Geometry: final body of the model. Coordinates: model frame, mm. Coordinates: 2 decimals unless noted, no trailing zeros. Write each loop counter-clockwise with the first axis right and the second up, starting at its lowest first coordinate (ties: lowest second). Pieces come first, ordered by that corner, then holes. Notation, with made-up numbers: (-19, 44.25) - (22, 44.25) arc R32 cw to (22, 81.25) - close; hole circle Ø6 at (51.5, 54.5). An arc over 180 degrees is marked (long way). Put each result on its own line as item: value.
Autodesk Inventor part; units mm, degrees
ref_plane "YZ Plane" through (0, 0, 0) normal (1, 0, 0) x (0, 1, 0)
ref_plane "XZ Plane" through (0, 0, 0) normal (0, 1, 0) x (-1, 0, 0)
ref_plane "XY Plane" through (0, 0, 0) normal (0, 0, 1) x (1, 0, 0)
sketch "Sketch1" plane through (0, 0, 0) normal (0, 0, 1) x (1, 0, 0)
  line L0 (-114.3, 77.8543) -> (-127, 77.8543)
  line L1 (-127, 77.8543) -> (-163.2323, 36.0005)
  arc A0 (-163.2323, 36.0005) -> (-215.9, -105.3078) centre (0, -105.3078) ccw
  line L2 (-152.4, -105.3078) -> (-215.9, -105.3078)
  arc A1 (152.4, -105.3078) -> (-152.4, -105.3078) centre (0, -105.3078) ccw
  line L3 (215.9, -105.3078) -> (152.4, -105.3078)
  arc A2 (215.9, -105.3078) -> (163.2323, 36.0005) centre (0, -105.3078) ccw
  line L4 (163.2323, 36.0005) -> (127, 77.8543)
  line L5 (127, 77.8543) -> (114.3, 77.8543)
  line L6 (114.3, 77.8543) -> (114.3, 90.5543)
  line L7 (114.3, 90.5543) -> (46.5518, 105.5138)
  arc A3 (46.5518, 105.5138) -> (-46.5518, 105.5138) centre (0, -105.3078) ccw
  line L8 (-46.5518, 105.5138) -> (-114.3, 90.5543)
  line L9 (-114.3, 90.5543) -> (-114.3, 77.8543)
  circle A4 centre (-174.6359, -42.9949) radius 3.302
  circle A5 centre (-181.5133, -67.4461) radius 3.302
  circle A6 centre (-184.9846, -92.6078) radius 3.302
  circle A7 centre (-12.7, 63.1241) radius 3.302
  circle A8 centre (-37.8617, 76.2055) radius 3.302
  circle A9 centre (-62.0706, 51.784) radius 3.302
  circle A10 centre (12.7, 63.1241) radius 3.302
  circle A11 centre (62.0706, 51.784) radius 3.302
  circle A12 centre (62.3129, 69.3281) radius 3.302
  circle A13 centre (174.6359, -42.9949) radius 3.302
  circle A14 centre (164.6231, -67.4949) radius 3.302
  circle A15 centre (181.5133, -67.4461) radius 3.302
  circle A16 centre (184.9846, -92.6078) radius 3.302
  circle A17 centre (168.4319, -92.6078) radius 3.302
  circle A18 centre (157.0918, -43.2372) radius 3.302
  circle A19 centre (37.8617, 76.2055) radius 3.302
  circle A20 centre (37.8128, 59.3154) radius 3.302
  circle A21 centre (12.7, 79.6768) radius 3.302
  circle A22 centre (-62.3129, 69.3281) radius 3.302
  circle A23 centre (-37.8128, 59.3154) radius 3.302
  circle A24 centre (-12.7, 79.6768) radius 3.302
  circle A25 centre (-168.4319, -92.6078) radius 3.302
  circle A26 centre (-164.6231, -67.4949) radius 3.302
  circle A27 centre (-157.0918, -43.2372) radius 3.302
  line L10 (-127, 143.7166) -> (-127, -105.3078)
  line L11 (-127, -21.0655) -> (-127, 108.4537)
  line L12 (-142.24, -21.0655) -> (-142.24, 38.6612) construction
  circle A28 centre (-142.24, -7.2274) radius 3.302
  circle A29 centre (-142.24, 18.1726) radius 3.302
  line L13 (-157.48, -21.0655) -> (-157.48, 42.6453)
  line L14 (-127, -21.0655) -> (-157.48, -21.0655)
  line L15 (-127, 108.4537) -> (-131.3752, 105.9825)
  line L16 (-143.2518, 91.0321) -> (-157.48, 42.6453)
  arc A30 (-131.3752, 105.9825) -> (-143.2518, 91.0321) centre (-118.8834, 83.8665) ccw
  circle A31 centre (142.24, 14.8706) radius 3.302
  circle A32 centre (-142.24, 14.8706) radius 3.302
  circle A33 centre (-142.24, -10.5294) radius 3.302
  circle A34 centre (142.24, -10.5294) radius 3.302
  point P0 (0, 0)
  dimension "d1" = 6.604
  dimension "d2" = 6.604
  dimension "d3" = 25.4
  dimension "d6" = 15.24
  dimension "d7" = 15.24
  dimension "d8" = 25.4
extrude "Extrusion1" add sketch "Sketch1" along normal blind 3.175 contours L10 L14 L13 L1 | L1 L16 A30 L15 L10 | A28 A33 | A29 A32 picked at (-142.4059, -12.7065) picked at (-142.4059, 12.6935)
sketch "Sketch2" plane through (0, 0, 0) normal (0, 0, -1) x (-1, 0, 0)
  line L0 (127, -21.0655) -> (127, 108.4537)
  line L1 (157.48, 42.6453) -> (157.48, -21.0655)
  line L2 (127, -21.0655) -> (157.48, -21.0655)
  line L3 (157.48, -21.0655) -> (157.48, -15.2234)
  line L4 (157.48, -15.2234) -> (127, -15.2234)
  line L5 (127, -15.2234) -> (127, -21.0655)
  point P0 (0, 0)
extrude "Extrusion2" cut sketch "Sketch2" against normal blind 25.4
properties part number "16in coil holder plate" material "UHMW, Black"
1. Ray query, probe 1 along Y at (x, z) = (-142.24, 1.45); probe 2 along Y at (x, z) = (-140, 0.75); probe 3 along X at (y, z) = (75.5, 0.8). Return the intervals inside material, ascending. Write a range as from..to.
Answer below:
probe 1: y = -15.22..-10.53, -3.93..14.87, 21.47..93.85
probe 2: y = -15.22..-9.65, -4.8..15.75, 20.6..97.98
probe 3: x = -147.82..-127
2. Mould query, pull axis X, two halves, no side actions, for faces 1 (the flat face through (-127, 47, 2)), 2 (the cylindrical face through (-145.54, 18.03, 1.57)), 3 (the flat face through (-142, -15.223, 2)), 4 (the flat face through (-129.157, 107.235, 1.565)). Classes: +X half, -X half, draft (parallel to the pull), parting line (faces both ways), or undercut.
Answer below:
face 1: +X half
face 2: undercut
face 3: draft
face 4: -X half
3. Section query A-A (z = 1.3). Return loops of the section in (x, y).
Answer below:
outline: (-157.48, -15.22) - (-127, -15.22) - (-127, 108.45) - (-131.38, 105.98) arc R25.4 ccw to (-143.25, 91.03) - (-157.48, 42.65) - close; hole circle Ø6.6 at (-142.24, -7.23); hole circle Ø6.6 at (-142.24, 18.17)
4. Section query B-B (y = 71). Return loops of the section in (x, z) (3 decimals), then the cut area to 3 significant figures.
Answer below:
outline: (-149.142, 0) - (-127, 0) - (-127, 3.175) - (-149.142, 3.175) - close
area: 70.3 mm²
5. Section query C-C (x = -147). Return loops of the section in (y, z) (3 decimals).
Answer below:
outline: (-15.223, 0) - (78.285, 0) - (78.285, 3.175) - (-15.223, 3.175) - close
6. Pin query (flat end, axial travel): pin 1 Ø7.5 at (x, y) = (-142.24, -7.23) entering from +Z (3 decimals); pin 2 Ø1.5 at (x, z) = (-138.5, 0.5) entering from +Y; pin 3 Ø1.5 at (y, z) = (53.5, 0.5) entering from -X. Return the tip coordinate at first contact, or that it passes through.
Answer below:
pin 1: stops at z = 3.175
pin 2: stops at y = 100.87
pin 3: stops at x = -154.51
